```python
from build123d import *

# Parameters (mm, degrees)
ESQUISSE1_W                = 580
ESQUISSE1_H                = 183
BOSS_EXTRU_1_DEPTH         = 10
ESQUISSE3_R                = 14
ESQUISSE3_R_2              = 10
ENL_V_MAT_EXTRU_1_DEPTH    = 10
R_P_TITION_LIN_AIRE1_COUNT = 2
R_P_TITION_LIN_AIRE1_PITCH = 280
CONG_1_R                   = 4


with BuildPart() as part:
    # Esquisse1 → Boss.-Extru.1 (new body)
    with BuildSketch(Plane.XY):
        with Locations((290, 91.5)):
            Rectangle(ESQUISSE1_W, ESQUISSE1_H)
    extrude(amount=BOSS_EXTRU_1_DEPTH)

    # Esquisse3 → Enlèv. mat.-Extru.1 (cut)
    with BuildSketch(Plane(origin=(0, 0, 0), x_dir=(-1, 0, 0), z_dir=(0, 0, -1))):
        with Locations((-201.25, 67)):
            Circle(ESQUISSE3_R)
        with Locations((-71.25, 106)):
            Circle(ESQUISSE3_R_2)
        with Locations((-166.25, 76)):
            Circle(ESQUISSE3_R)
        with Locations((-135, 94)):
            Circle(ESQUISSE3_R)
        with Locations((-237.25, 106)):
            Circle(ESQUISSE3_R)
        with Locations((-201.25, 106)):
            Circle(ESQUISSE3_R)
        with Locations((-166.25, 115)):
            Circle(ESQUISSE3_R)
        with Locations((-135, 133)):
            Circle(ESQUISSE3_R)
    enl_v_mat_extru_1 = extrude(amount=-ENL_V_MAT_EXTRU_1_DEPTH, mode=Mode.SUBTRACT)

    # Répétition linéaire1: Enlèv. mat.-Extru.1 ×2
    with Locations(*[(i * R_P_TITION_LIN_AIRE1_PITCH, 0, 0) for i in range(1, R_P_TITION_LIN_AIRE1_COUNT)]):
        add(enl_v_mat_extru_1, mode=Mode.SUBTRACT)

    # Congé1
    cong_1_edges = [part.edges().sort_by_distance(p)[0] for p in [
        (290, 183, 0),
    ]]
    fillet(cong_1_edges, radius=CONG_1_R)


solid = part.part
```
CAD build for the part. Positions are in the model's coordinates, mm. Coordinates: 2 decimals unless noted, no trailing zeros. Order: outer loops, then holes, each group sorted by start corner. A loop starts at its lowest first (then second) coordinate and runs counter-clockwise, first axis right, second up. Notation, with made-up numbers: (22.5, 85.5) -> (72.5, 85.5) arc R22 ccw to (72.5, 97.5) -> close; hole circle Ø1 at (21, 56). An arc over 180 degrees is marked (long way). Use one line per item in the form item = value. Start each with the question number.
1) Band-saw the part on C-C on y = 140.5. Give the cut face in (x, z), then the cut area to 3 significant figures.
2) Drill centre lines: L1, parallel to Y at x = 135, z = 7; L2, parallel to Y at x = 166.25, z = 4; L3, parallel to Y at x = 237.25, z = 5.75. Where is each one in solid material? Low to high. Write a range as [from, to].
3) Band-saw the part on D-D on x = 71.25. Give the cut face in (y, z), then the cut area to 3 significant figures.
4) Band-saw the part on A-A on x = 201.25. Give the cut face in (y, z), then the cut area to 3 significant figures.
5) Pull direction Y, two halves, no side cores. Call faces 1 (the flat face through (286, 0, 5)), 2 (the cylindrical face through (136.82, 146.88, 4.93)), 3 (the cylindrical face through (432.9, 80.21, 4.93)), 4 (the flat face through (286, 91, 0)): +Y half, -Y half, draft (parallel to the pull), parting line (faces both ways), or undercut.
6) Band-saw the part on B-B on z = 6.75. State how many separate pieces and enclosed holes the cut face has, then the cut area to 3 significant figures.
Entries:
q1.outline = (0, 0) -> (123.18, 0) -> (123.18, 10) -> (0, 10) -> close; (146.82, 0) -> (403.18, 0) -> (403.18, 10) -> (146.82, 10) -> close; (426.82, 0) -> (580, 0) -> (580, 10) -> (426.82, 10) -> close
q1.area = 5,330 mm2
q2.L1 = [0, 80], [108, 119], [147, 183]
q2.L2 = [0, 62], [90, 101], [129, 183]
q2.L3 = [0, 92], [120, 183]
q3.outline = (0, 0) -> (96, 0) -> (96, 10) -> (0, 10) -> close; (116, 0) -> (179, 0) arc R4 ccw to (183, 4) -> (183, 10) -> (116, 10) -> close
q3.area = 1,630 mm2
q4.outline = (0, 0) -> (53, 0) -> (53, 10) -> (0, 10) -> close; (81, 0) -> (92, 0) -> (92, 10) -> (81, 10) -> close; (120, 0) -> (179, 0) arc R4 ccw to (183, 4) -> (183, 10) -> (120, 10) -> close
q4.area = 1,270 mm2
q5.face_1 = -Y half
q5.face_2 = undercut
q5.face_3 = undercut
q5.face_4 = draft
q6.separate_pieces = 1
q6.enclosed_holes = 16
q6.area = 96,900 mm2
